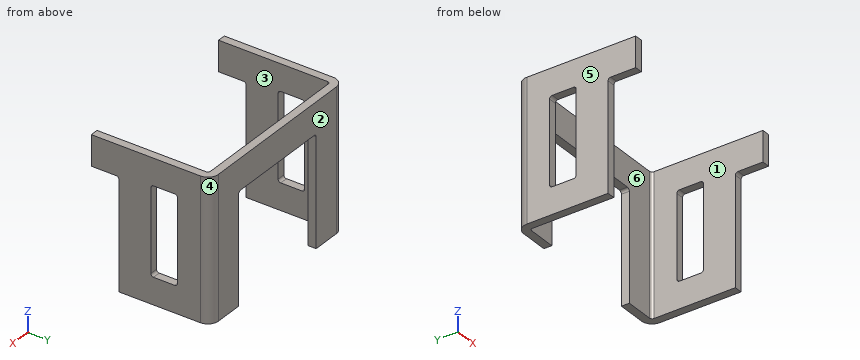
```python
from build123d import *

# Parameters (mm, degrees)
SKETCH1_W           = 35
SKETCH1_H           = 26.5
BOSS_EXTRUDE1_DEPTH = 22.5
SKETCH2_W           = 32
SKETCH2_H           = 21
CUT_EXTRUDE1_DEPTH  = 27.5
SKETCH3_W           = 20.8
SKETCH3_H           = 5.2
CUT_EXTRUDE2_DEPTH  = 2.5
SKETCH4_W           = 20.4
SKETCH4_H           = 20.7
CUT_EXTRUDE3_DEPTH  = 2.5
SKETCH5_W           = 20.8
SKETCH5_H           = 5.2
CUT_EXTRUDE4_DEPTH  = 2.5
FILLET1_R           = 0.5
FILLET2_R           = 2
SKETCH6_W           = 16.5
SKETCH6_H           = 5
CUT_EXTRUDE5_DEPTH  = 35
FILLET3_R           = 0.5


with BuildPart() as part:
    # Sketch1 → Boss-Extrude1 (new body)
    with BuildSketch(Plane(origin=(0, 14, 0), x_dir=(1, 0, 0), z_dir=(0, 1, 0))):
        with Locations((0, -2.75)):
            Rectangle(SKETCH1_W, SKETCH1_H)
    extrude(amount=-BOSS_EXTRUDE1_DEPTH)

    # Sketch2 → Cut-Extrude1 (cut, through all)
    with BuildSketch(Plane.XY.offset(16)):
        with Locations((0, 2)):
            Rectangle(SKETCH2_W, SKETCH2_H)
    extrude(amount=-CUT_EXTRUDE1_DEPTH, mode=Mode.SUBTRACT)

    # Sketch3 → Cut-Extrude2 (cut, through all)
    with BuildSketch(Plane.ZY.offset(-16)):
        with Locations((-0.1, -5.9)):
            Rectangle(SKETCH3_W, SKETCH3_H)
    extrude(amount=-CUT_EXTRUDE2_DEPTH, mode=Mode.SUBTRACT)

    # Sketch4 → Cut-Extrude3 (cut, through all)
    with BuildSketch(Plane.XZ.offset(-12.5)):
        with Locations((0, -0.15)):
            Rectangle(SKETCH4_W, SKETCH4_H)
    extrude(amount=-CUT_EXTRUDE3_DEPTH, mode=Mode.SUBTRACT)

    # Sketch5 → Cut-Extrude4 (cut, through all)
    with BuildSketch(Plane(origin=(-16, 0, 0), x_dir=(0, 0, -1), z_dir=(1, 0, 0))):
        with Locations((0.1, -5.9)):
            Rectangle(SKETCH5_W, SKETCH5_H)
    extrude(amount=-CUT_EXTRUDE4_DEPTH, mode=Mode.SUBTRACT)

    # Fillet1
    fillet1_edges = [part.edges().sort_by_distance(p)[0] for p in [
        (-16, 12.5, 2.75),
        (16, 12.5, 2.75),
    ]]
    fillet(fillet1_edges, radius=FILLET1_R)

    # Fillet2
    fillet2_edges = [part.edges().sort_by_distance(p)[0] for p in [
        (-17.5, 14, 2.75),
        (17.5, 14, 2.75),
    ]]
    fillet(fillet2_edges, radius=FILLET2_R)

    # Sketch6 → Cut-Extrude5 (cut)
    with BuildSketch(Plane(origin=(17.5, 0, 0), x_dir=(0, 0, -1), z_dir=(1, 0, 0))):
        with Locations((-2.75, 5.2)):
            Rectangle(SKETCH6_W, SKETCH6_H)
    extrude(amount=-CUT_EXTRUDE5_DEPTH, mode=Mode.SUBTRACT)

    # Fillet3
    fillet3_edges = [part.edges().sort_by_distance(p)[0] for p in [
        (-16.75, 2.7, 11),
        (16.75, 2.7, 11),
        (-16.75, 7.7, 11),
        (16.75, 7.7, 11),
        (-16.75, 7.7, -5.5),
        (16.75, 7.7, -5.5),
        (-16.75, 2.7, -5.5),
        (16.75, 2.7, -5.5),
        (16.75, -3.3, 10.3),
        (-10.2, 13.25, 10.2),
        (10.2, 13.25, 10.2),
        (-16.75, -3.3, 10.3),
    ]]
    fillet(fillet3_edges, radius=FILLET3_R)


solid = part.part
```
Geometry: final body of the model. Coordinates: model frame, mm. Face numbers are marked on the shaded views. A direction names the side the tool comes from. Coordinates: 2 decimals unless noted, no trailing zeros. Order: outer loops, then holes, each group sorted by start corner. A loop starts at its lowest first (then second) coordinate and runs counter-clockwise, first axis right, second up. Notation, with made-up numbers: (-5, -37) -> (29, -37) arc R28 ccw to (29, -16) -> close; hole circle Ø1 at (64, 15.25). An arc over 180 degrees is marked (long way). Write each question's results on one line, items separated by ' | '. Start each with the question number.
1) First-contact query: pin 1 (1.6 mm diameter, centred on x = -17, z = 3, fed in from -Y); pin 2 (1.2 mm diameter, centred on x = -17, z = 3.5, fed in from +Y); pin 3 (5 mm diameter, centred on x = 11, z = -4, fed in from -Y). Flat tips, straight axial feed; report the tip coordinate or a pass-through.
2) Set-up query: the marked faces 1 and 2. Return all of +Z, -Z, +X, -X, +Y, -Y with unobstructed straight access to the full face (end or side cutting, diameter ignored); none if empty.
3) Cut plane A-A, the plane z = -7.75. Output: boundary loops of the cut face in (x, y), and give its area (3 significant figures).
4) Cut plane C-C, the plane z = 5. Output: boundary loops of the cut face in (x, y), and give its area (3 significant figures).
5) Cut plane D-D, the plane x = 14.5. Output: boundary loops of the cut face in (y, z).
6) Cut plane B-B, the plane y = 9. Output: boundary loops of the cut face in (x, z).
7) Material intervals for line 1 along X through (y, z) = (3.75, -9.25); line 2 along Y through (x, z) = (13, -0.25), sorted ascending.
8) Mould query, pull axis X, two halves, no side actions, for the marked faces 3, 4, 5 and 6. Classes: released by +X, released by -X, zero draft, split by the parting line, or undercut.
Checks:
1) pin 1: y = -3.3 | pin 2: y = 13.79 | pin 3: y = 12.5
2) face 1: +Z, -Z, -Y | face 2: +Z, -Z, +X, -X, +Y
3) outline: (-17.5, -3.3) -> (-16, -3.3) -> (-16, 12) arc R0.5 cw to (-15.5, 12.5) -> (-10.2, 12.5) -> (-10.2, 14) -> (-15.5, 14) arc R2 ccw to (-17.5, 12) -> close; (10.2, 12.5) -> (15.5, 12.5) arc R0.5 cw to (16, 12) -> (16, -3.3) -> (17.5, -3.3) -> (17.5, 12) arc R2 ccw to (15.5, 14) -> (10.2, 14) -> close | area: 67.7 mm^2
4) outline: (-17.5, -3.3) -> (-16, -3.3) -> (-16, 2.7) -> (-17.5, 2.7) -> close; (-17.5, 7.7) -> (-16, 7.7) -> (-16, 12) arc R0.5 cw to (-15.5, 12.5) -> (-10.2, 12.5) -> (-10.2, 14) -> (-15.5, 14) arc R2 ccw to (-17.5, 12) -> close; (10.2, 12.5) -> (15.5, 12.5) arc R0.5 cw to (16, 12) -> (16, 7.7) -> (17.5, 7.7) -> (17.5, 12) arc R2 ccw to (15.5, 14) -> (10.2, 14) -> close; (16, -3.3) -> (17.5, -3.3) -> (17.5, 2.7) -> (16, 2.7) -> close | area: 52.7 mm^2
5) outline: (12.5, -10.5) -> (14, -10.5) -> (14, 16) -> (12.5, 16) -> close
6) outline: (-17.5, -10.5) -> (-16, -10.5) -> (-16, 16) -> (-17.5, 16) -> close; (16, -10.5) -> (17.5, -10.5) -> (17.5, 16) -> (16, 16) -> close
7) line 1: -17.5 to -16, 16 to 17.5 | line 2: 12.5 to 14
8) face 3: undercut | face 4: released by +X | face 5: released by -X | face 6: undercut
